from build123d import *

# Parameters (mm, degrees)
SKETCH_1_R      = 3
SKETCH_1_R_2    = 1.6
EXTRUDE_1_DEPTH = 19.325


# Read off the part's stored shape, not the designer's step: M3x0.5 ねじ穴1
with BuildPart() as part:
    # ｽｹｯﾁ1 → ﾎﾞｽ - 押し出し1 (new, symmetric)
    # profile 1 of 2: a face of its own
    with BuildSketch(Plane.XY):
        Circle(SKETCH_1_R)
        Circle(SKETCH_1_R_2, mode=Mode.SUBTRACT)
    # profile 2 of 2: a face of its own
    with BuildSketch(Plane.XY):
        Circle(SKETCH_1_R_2)
    extrude(amount=EXTRUDE_1_DEPTH, both=True)

    # M3x0.5 ねじ穴1 outline → M3x0.5 ねじ穴1 (revolve, cut)
    with BuildSketch(Plane.XZ):
        Polygon((1.25, -10.825), (0, -10.073924226), (0, -19.325), (1.25, -19.325), align=None)
        Polygon((0, 19.325), (0, 10.073924226), (1.25, 10.825), (1.25, 19.325), align=None)
    revolve(axis=Axis((0, 0, 0), (0, 0, 1)), mode=Mode.SUBTRACT)


solid = part.part
Input: part model. Units: mm. Frame: model coordinates. A direction names the side the tool comes from. Round coordinates to 2 decimals unless told otherwise and drop trailing zeros. Write each loop counter-clockwise with the first axis right and the second up, starting at its lowest first coordinate (ties: lowest second). Pieces come first, ordered by that corner, then holes.
1) Ray query, L1, parallel to Y at x = 0, z = -14.5; L2, parallel to Y at x = -0.5, z = -13.5. Return the intervals inside material, ascending.
2) Cut plane A-A (z = 6). Return the cut outline in (x, y).
3) Reachability of faces 1 (the cylindrical face through (-0.27, -1.22, 15.13)), 2 (the conical face through (0.19, 0.06, -10.194)) from +Z, -Z, +X, -X, +Y, -Y: full face, straight path, thin tool, end or side. Return the list, or none.
4) Cut plane B-B (x = 2.4). Return the cut outline in (y, z) (3 decimals).
5) Draft query along X for faces 3 (the cylindrical face through (-3, 0, 0)), 4 (the flat face through (1, -1, -19.325)), 5 (the cylindrical face through (-0.27, -1.22, -15.02)). Return one class per face: pulls with the +X half, pulls with the -X half, needs draft (parallel to the pull), parting line crosses it, or undercut.
6) Cut plane C-C (y = -2.1). Return the cut outline in (x, z) (3 decimals).
Geometry says:
1. L1: y = -3 to -1.25, 1.25 to 3
1. L2: y = -2.96 to -1.15, 1.15 to 2.96
2. outline: circle Ø6 at (0, 0)
3. face 1: +Z
3. face 2: -Z
4. outline: (-1.8, -19.325) - (1.8, -19.325) - (1.8, 19.325) - (-1.8, 19.325) - close
5. face 3: parting line crosses it
5. face 4: needs draft
5. face 5: undercut
6. outline: (-2.142, -19.325) - (2.142, -19.325) - (2.142, 19.325) - (-2.142, 19.325) - close
